Source: CAD feature listing. Evaluate the final solid. Frame: model axes, mm. Round coordinates to 2 decimals unless told otherwise and drop trailing zeros. Write each loop counter-clockwise with the first axis right and the second up, starting at its lowest first coordinate (ties: lowest second). Pieces come first, ordered by that corner, then holes. Notation, with made-up numbers: (73.5, -31) -> (94.5, -31) arc R21 cw to (94.5, -20) -> close; hole circle Ø5 at (8.25, -10.75). An arc over 180 degrees is marked (long way). Return JSON: item names as keys, results as strings. Group by question number.
from build123d import *

# Parameters (mm, degrees)
ESQUISSE1_W             = 11.5
ESQUISSE1_H             = 2
EXTRU_MINCE1_DEPTH      = 50
ESQUISSE2_R             = 1.5
ENL_V_MAT_EXTRU_1_DEPTH = 3
CONG_1_R                = 5


with BuildPart() as part:
    # Esquisse1 → Extru.-Mince1 (new body)
    with BuildSketch(Plane.XY):
        with Locations((5.75, 1)):
            Rectangle(ESQUISSE1_W, ESQUISSE1_H)
    extrude(amount=EXTRU_MINCE1_DEPTH)

    # Esquisse2 → Enlèv. mat.-Extru.1 (cut)
    with BuildSketch(Plane(origin=(0, 2, 0), x_dir=(1, 0, 0), z_dir=(0, 1, 0))):
        with Locations(Location((5.75, -6, 0), (0, 0, 270))):
            Circle(ESQUISSE2_R)
        with Locations(Location((5.75, -27.56965461, 0), (0, 0, 270))):
            Circle(ESQUISSE2_R)
        with Locations(Location((5.75, -44, 0), (0, 0, 270))):
            Circle(ESQUISSE2_R)
    extrude(amount=-ENL_V_MAT_EXTRU_1_DEPTH, mode=Mode.SUBTRACT)

    # Congé1
    cong_1_edges = [part.edges().sort_by_distance(p)[0] for p in [
        (0, 1, 50),
        (0, 1, 0),
        (11.5, 1, 0),
        (11.5, 1, 50),
    ]]
    fillet(cong_1_edges, radius=CONG_1_R)


solid = part.part
Item 1: First-contact query: pin 1 Ø1.8 at (x, z) = (5.75, 27.57) entering from +Y. Flat tip, straight axial feed; report the tip coordinate or a pass-through.
Item 2: Cut plane A-A on y = 0.95. Output: boundary loops of the cut face in (x, z), and give its area (3 significant figures).
Item 3: Cut plane B-B on z = 6. Output: boundary loops of the cut face in (x, y), and give its area (3 significant figures).
Item 4: Cut plane D-D on x = 3. Output: boundary loops of the cut face in (y, z).
Item 5: Material intervals for probe 1 along X at (y, z) = (1.2, 6); probe 2 along Z at (x, y) = (7, 0.75); probe 3 along Z at (x, y) = (5, 1.3), sorted ascending.
Item 6: Cut plane C-C on x = 5.75. Output: boundary loops of the cut face in (y, z).
Item 7: Pull-direction query (Z, two-part tool) for faces 1 (the cylindrical face through (1, 1, 48)), 2 (the cylindrical face through (6.2, 1, 29)), 3 (the flat face through (0, 1, 25)), 4 (the cylindrical face through (5.8, 1, 42.5)); classes: +Z half, -Z half, draft (parallel to the pull), parting line (faces both ways), or undercut.
Here are the results:
{
 "1": {"pin 1": "passes through"},
 "2": {"outline": "(0, 5) arc R5 ccw to (5, 0) -> (6.5, 0) arc R5 ccw to (11.5, 5) -> (11.5, 45) arc R5 ccw to (6.5, 50) -> (5, 50) arc R5 ccw to (0, 45) -> close; hole circle Ø3 at (5.75, 6); hole circle Ø3 at (5.75, 27.57); hole circle Ø3 at (5.75, 44)", "area": "532 mm^2"},
 "3": {"outline": "(0, 0) -> (4.25, 0) -> (4.25, 2) -> (0, 2) -> close; (7.25, 0) -> (11.5, 0) -> (11.5, 2) -> (7.25, 2) -> close", "area": "17.0 mm^2"},
 "4": {"outline": "(0, 0.42) -> (2, 0.42) -> (2, 49.58) -> (0, 49.58) -> close"},
 "5": {"probe 1": "x = 0 to 4.25, 7.25 to 11.5", "probe 2": "z = 0.03 to 5.17, 6.83 to 26.74, 28.4 to 43.17, 44.83 to 49.97", "probe 3": "z = 0 to 4.7, 7.3 to 26.27, 28.87 to 42.7, 45.3 to 50"},
 "6": {"outline": "(0, 0) -> (2, 0) -> (2, 4.5) -> (0, 4.5) -> close; (0, 7.5) -> (2, 7.5) -> (2, 26.07) -> (0, 26.07) -> close; (0, 29.07) -> (2, 29.07) -> (2, 42.5) -> (0, 42.5) -> close; (0, 45.5) -> (2, 45.5) -> (2, 50) -> (0, 50) -> close"},
 "7": {"face 1": "+Z half", "face 2": "undercut", "face 3": "draft", "face 4": "undercut"}
}
